from build123d import *

# Parameters (mm, degrees)
SKETCH1_R                  = 6
BEARING_JOURNAL_12MM_DEPTH = 19.9
SKETCH2_R                  = 7
BOSS_EXTRUDE2_DEPTH        = 5
SKETCH3_R                  = 12.5
BODY_M25_DEPTH             = 65
SKETCH4_R                  = 1.714870996
CABLE_DEPTH                = 25
SKETCH5_R                  = 3
CUT_EXTRUDE_M6_DEPTH       = 10


with BuildPart() as part:
    # Sketch1 → Bearing Journal-12mm (new body)
    with BuildSketch(Plane.XY):
        with Locations(Location((0, 0, 0), (0, 0, 180))):
            Circle(SKETCH1_R)
    extrude(amount=BEARING_JOURNAL_12MM_DEPTH)

    # Sketch2 → Boss-Extrude2 (add)
    with BuildSketch(Plane.XY.offset(19.9)):
        Circle(SKETCH2_R)
    extrude(amount=BOSS_EXTRUDE2_DEPTH)

    # Sketch3 → Body-M25 (add)
    with BuildSketch(Plane.XY.offset(24.9)):
        Circle(SKETCH3_R)
    extrude(amount=BODY_M25_DEPTH)

    # Sketch4 → Cable (add)
    with BuildSketch(Plane.XY.offset(89.9)):
        Circle(SKETCH4_R)
    extrude(amount=CABLE_DEPTH)

    # Sketch5 → Cut-Extrude M6 (cut)
    with BuildSketch(Plane(origin=(0, 0, 0), x_dir=(-1, 0, 0), z_dir=(0, 0, -1))):
        Circle(SKETCH5_R)
    extrude(amount=-CUT_EXTRUDE_M6_DEPTH, mode=Mode.SUBTRACT)


solid = part.part
CAD build for the part. Positions are in the model's coordinates, mm. A direction names the side the tool comes from. Round coordinates to 2 decimals unless told otherwise and drop trailing zeros. Write each loop counter-clockwise with the first axis right and the second up, starting at its lowest first coordinate (ties: lowest second). Pieces come first, ordered by that corner, then holes.
(1) Drop flat-ended pins along their axis: P1, Ø1.8, axis at x = 0, y = 1, coming from the -Z side; P2, Ø4, axis at x = -9.5, y = 7, coming from the +Z side; P3, Ø6, axis at y = -5, z = 18.5, coming from the +X side. Give the stop position or say it passes through.
(2) 3-axis set-ups, long thin cutter, end or side, ignore diameter. For faces 1 (the face through (3, 1, 0)), 2 (the face through (6.466, -2.681, 22.365)), 3 (the face through (-0.372, -1.674, 102.225)): which of +Z, -Z, +X, -X, +Y, -Y reach the whole face in a straight line?
(3) Probe line 1 along Y through (x, z) = (0, 6.5); line 2 along Z through (x, y) = (-7.5, 0.25); line 3 along Z through (x, y) = (-0.75, 6). List the from-to ranges inside material, lowest first.
(4) Slice it at D-D, the plane y = -4.5. Write the cut outline in (x, z), and give its area (3 significant figures).
(5) Mould opens along Y. For faces 4 (the face through (11.923, 3.755, 56.945)), 5 (the face through (0, 0, 10)), 6 (the face through (6, 2, 19.9)), 7 (the face through (3, 0, 5)) say: pulls with the +Y half, pulls with the -Y half, needs draft (parallel to the pull), parting line crosses it, or undercut.
(6) Slice it at C-C, the plane z = 47.5. Write the cut outline in (x, y), and give its area (3 significant figures).
(7) Slice it at A-A, the plane y = 0. Write the cut outline in (x, z), and give its area (3 significant figures).
From the geometry:
1. P1: stops at z = 10
1. P2: stops at z = 89.9
1. P3: stops at x = 6.59
2. face 1: -Z, +X, -X, +Y, -Y
2. face 2: -Z
2. face 3: +Z
3. line 1: y = -6 to -3, 3 to 6
3. line 2: z = 24.9 to 89.9
3. line 3: z = 19.9 to 89.9
4. outline: (-11.66, 24.9) - (-5.36, 24.9) - (-5.36, 19.9) - (-3.97, 19.9) - (-3.97, 0) - (3.97, 0) - (3.97, 19.9) - (5.36, 19.9) - (5.36, 24.9) - (11.66, 24.9) - (11.66, 89.9) - (-11.66, 89.9) - close
4. area: 1,730 mm2
5. face 4: parting line crosses it
5. face 5: undercut
5. face 6: needs draft
5. face 7: undercut
6. outline: circle Ø25 at (0, 0)
6. area: 491 mm2
7. outline: (-12.5, 24.9) - (-7, 24.9) - (-7, 19.9) - (-6, 19.9) - (-6, 0) - (-3, 0) - (-3, 10) - (3, 10) - (3, 0) - (6, 0) - (6, 19.9) - (7, 19.9) - (7, 24.9) - (12.5, 24.9) - (12.5, 89.9) - (1.71, 89.9) - (1.71, 114.9) - (-1.71, 114.9) - (-1.71, 89.9) - (-12.5, 89.9) - close
7. area: 1,960 mm2
